```python
from build123d import *

# Parameters (mm, degrees)
SKETCH1_W                                   = 80
SKETCH1_H                                   = 60
BOSS_EXTRUDE1_DEPTH                         = 100
CUT_EXTRUDE1_START                          = 5
SKETCH2_W                                   = 35
SKETCH2_H                                   = 55
CUT_EXTRUDE1_DEPTH                          = 95
SKETCH3_W                                   = 80
SKETCH3_H                                   = 5
BOSS_EXTRUDE2_DEPTH                         = 70
BOSS_EXTRUDE3_DEPTH                         = 10
SKETCH5_W                                   = 22.5
SKETCH5_H                                   = 2.5
SKETCH5_W_2                                 = 20
CUT_EXTRUDE2_DEPTH                          = 7.5
SKETCH6_W                                   = 35
SKETCH6_H                                   = 12
CUT_EXTRUDE4_DEPTH                          = 57.5
CUT_EXTRUDE6_REACH                          = 184.483
SKETCH7_R                                   = 4
SKETCH9_W                                   = 80
SKETCH9_H                                   = 50
BOSS_EXTRUDE4_DEPTH                         = 5
SKETCH11_W                                  = 75
SKETCH11_H                                  = 32.5
CUT_EXTRUDE7_DEPTH                          = 2
SKETCH13_W                                  = 6
SKETCH13_H                                  = 6
CUT_EXTRUDE8_DEPTH                          = 166.90660023
BOSS_EXTRUDE5_DEPTH                         = 10
SKETCH15_W                                  = 6
SKETCH15_H                                  = 4
BOSS_EXTRUDE6_DEPTH                         = 1
BOSS_EXTRUDE7_START                         = -2.5
SKETCH15_2_W                                = 6
SKETCH15_2_H                                = 4
BOSS_EXTRUDE7_DEPTH                         = 1
SKETCH17_W                                  = 6
SKETCH17_H                                  = 4
BOSS_EXTRUDE8_DEPTH                         = 1
SKETCH18_W                                  = 3
SKETCH18_H                                  = 4
CUT_EXTRUDE9_OLED_CABLE_DEPTH               = 154.430766146
SKETCH20_W                                  = 5
SKETCH20_H                                  = 5
CUT_EXTRUDE10_SOLENOID_WIRE_DEPTH           = 166.90660023
SKETCH21_W                                  = 2
SKETCH21_H                                  = 32
BOSS_EXTRUDE9_SOLENOID_SIDE_SUPPORT_DEPTH   = 13
BOSS_EXTRUDE12_SOLENOID_REAR_SUPPORT_DEPTH  = 2
SKETCH27_W                                  = 2.5
SKETCH27_H                                  = 50
BOSS_EXTRUDE13_SOLENOID_SECTION_WALLS_DEPTH = 15
SKETCH29_W                                  = 70
SKETCH29_H                                  = 5
SKETCH29_W_2                                = 110
BOSS_EXTRUDE14_GUIDE_DEPTH                  = 5
BOSS_EXTRUDE15_START                        = -80
SKETCH29_2_W                                = 70
SKETCH29_2_H                                = 5
SKETCH29_2_W_2                              = 110
BOSS_EXTRUDE15_DEPTH                        = 5
SKETCH30_W                                  = 110
SKETCH30_H                                  = 2.5
SKETCH30_W_2                                = 70
BOSS_EXTRUDE16_DEPTH                        = 2.5
BOSS_EXTRUDE17_START                        = -87.5
SKETCH30_2_W                                = 110
SKETCH30_2_H                                = 2.5
SKETCH30_2_W_2                              = 70
BOSS_EXTRUDE17_DEPTH                        = 2.5


with BuildPart() as part:
    # Sketch1 → Boss-Extrude1 (new body)
    with BuildSketch(Plane(origin=(0, 0, 0), x_dir=(1, 0, 0), z_dir=(0, 1, 0))):
        with Locations((40, 30)):
            Rectangle(SKETCH1_W, SKETCH1_H)
    extrude(amount=BOSS_EXTRUDE1_DEPTH)

    # Sketch2 → Cut-Extrude1 (cut)
    with BuildSketch(Plane(origin=(0, 0, 0), x_dir=(1, 0, 0), z_dir=(0, 1, 0)).offset(CUT_EXTRUDE1_START)):
        with Locations((20, 30)):
            Rectangle(SKETCH2_W, SKETCH2_H)
        with Locations((60, 30)):
            Rectangle(SKETCH2_W, SKETCH2_H)
    extrude(amount=CUT_EXTRUDE1_DEPTH, mode=Mode.SUBTRACT)

    # Sketch3 → Boss-Extrude2 (add)
    with BuildSketch(Plane.XY):
        with Locations((40, 2.5)):
            Rectangle(SKETCH3_W, SKETCH3_H)
    extrude(amount=BOSS_EXTRUDE2_DEPTH)

    # Sketch4 → Boss-Extrude3 (add)
    with BuildSketch(Plane(origin=(0, 5, 0), x_dir=(1, 0, 0), z_dir=(0, 1, 0))):
        Polygon((80, 0), (77.5, 0), (77.5, -67.5), (42.5, -67.5), (42.5, 0), (37.5, 0), (37.5, -67.5), (2.5, -67.5), (2.5, 0), (0, 0), (0, -70), (80, -70), align=None)
    extrude(amount=BOSS_EXTRUDE3_DEPTH)

    # Sketch5 → Cut-Extrude2 (cut)
    with BuildSketch(Plane(origin=(0, 15, 0), x_dir=(1, 0, 0), z_dir=(0, 1, 0))):
        with Locations((18.75, -68.75)):
            Rectangle(SKETCH5_W, SKETCH5_H)
        with Locations((60, -68.75)):
            Rectangle(SKETCH5_W_2, SKETCH5_H)
    extrude(amount=-CUT_EXTRUDE2_DEPTH, mode=Mode.SUBTRACT)

    # Sketch6 → Cut-Extrude4 (cut)
    with BuildSketch(Plane.XY):
        with Locations((20, 11)):
            Rectangle(SKETCH6_W, SKETCH6_H)
        with Locations((60, 11)):
            Rectangle(SKETCH6_W, SKETCH6_H)
    extrude(amount=-CUT_EXTRUDE4_DEPTH, mode=Mode.SUBTRACT)

    # Sketch7 → Cut-Extrude6 (cut, up to next)
    with BuildSketch(Plane(origin=(0, 0, -60), x_dir=(-1, 0, 0), z_dir=(0, 0, -1)), mode=Mode.PRIVATE) as cut_extrude6_sk1:
        with Locations((-20, 11.5)):
            Circle(SKETCH7_R)
    cut_extrude6_tool1 = extrude(cut_extrude6_sk1.sketch, amount=-CUT_EXTRUDE6_REACH, mode=Mode.PRIVATE) & part.part
    # Sketch7 → Cut-Extrude6 (cut, up to next)
    with BuildSketch(Plane(origin=(0, 0, -60), x_dir=(-1, 0, 0), z_dir=(0, 0, -1)), mode=Mode.PRIVATE) as cut_extrude6_sk2:
        with Locations((-60, 11.5)):
            Circle(SKETCH7_R)
    cut_extrude6_tool2 = extrude(cut_extrude6_sk2.sketch, amount=-CUT_EXTRUDE6_REACH, mode=Mode.PRIVATE) & part.part
    add(cut_extrude6_tool1.solids().sort_by_distance((20, 11.5, -60))[0], mode=Mode.SUBTRACT)
    add(cut_extrude6_tool2.solids().sort_by_distance((60, 11.5, -60))[0], mode=Mode.SUBTRACT)

    # Sketch9 → Boss-Extrude4 (add)
    with BuildSketch(Plane(origin=(0, 0, 0), x_dir=(1, 0, 0), z_dir=(0, 1, 0))):
        with Locations((40, 85)):
            Rectangle(SKETCH9_W, SKETCH9_H)
    extrude(amount=BOSS_EXTRUDE4_DEPTH)

    # Sketch11 → Cut-Extrude7 (cut)
    with BuildSketch(Plane.XZ):
        with Locations((40, 53.75)):
            Rectangle(SKETCH11_W, SKETCH11_H)
    extrude(amount=-CUT_EXTRUDE7_DEPTH, mode=Mode.SUBTRACT)

    # Sketch13 → Cut-Extrude8 (cut, through all)
    with BuildSketch(Plane(origin=(0, 5, 0), x_dir=(1, 0, 0), z_dir=(0, 1, 0))):
        with Locations((20, -64.5)):
            Rectangle(SKETCH13_W, SKETCH13_H)
        with Locations((60, -64.5)):
            Rectangle(SKETCH13_W, SKETCH13_H)
    extrude(amount=-CUT_EXTRUDE8_DEPTH, mode=Mode.SUBTRACT)

    # Sketch14 → Boss-Extrude5 (add)
    with BuildSketch(Plane.XY):
        Polygon((25, 100), (26, 100), (26, 71), (54, 71), (54, 100), (55, 100), (55, 70), (54, 70), (26, 70), (25, 70), align=None)
    extrude(amount=BOSS_EXTRUDE5_DEPTH)

    # Sketch15 → Boss-Extrude6 (add)
    with BuildSketch(Plane.XY.offset(10)):
        with Locations((28, 72)):
            Rectangle(SKETCH15_W, SKETCH15_H)
        with Locations((52, 72)):
            Rectangle(SKETCH15_W, SKETCH15_H)
    extrude(amount=-BOSS_EXTRUDE6_DEPTH)

    # Sketch15<2> → Boss-Extrude7 (add)
    with BuildSketch(Plane.XY.offset(10).offset(BOSS_EXTRUDE7_START)):
        with Locations((28, 72)):
            Rectangle(SKETCH15_2_W, SKETCH15_2_H)
        with Locations((52, 72)):
            Rectangle(SKETCH15_2_W, SKETCH15_2_H)
    extrude(amount=-BOSS_EXTRUDE7_DEPTH)

    # Sketch17 → Boss-Extrude8 (add)
    with BuildSketch(Plane.XY.offset(10)):
        with Locations((28, 98)):
            Rectangle(SKETCH17_W, SKETCH17_H)
        with Locations((52, 98)):
            Rectangle(SKETCH17_W, SKETCH17_H)
    extrude(amount=-BOSS_EXTRUDE8_DEPTH)

    # Sketch18 → Cut-Extrude9 (OLED Cable) (cut, through all)
    with BuildSketch(Plane(origin=(0, 71, 0), x_dir=(1, 0, 0), z_dir=(0, 1, 0))):
        with Locations((40, -2)):
            Rectangle(SKETCH18_W, SKETCH18_H)
    extrude(amount=-CUT_EXTRUDE9_OLED_CABLE_DEPTH, mode=Mode.SUBTRACT)

    # Sketch20 → Cut-Extrude10 (Solenoid Wire) (cut, through all)
    with BuildSketch(Plane(origin=(0, 5, 0), x_dir=(1, 0, 0), z_dir=(0, 1, 0))):
        with Locations((60, 62.5)):
            Rectangle(SKETCH20_W, SKETCH20_H)
        with Locations((20, 62.5)):
            Rectangle(SKETCH20_W, SKETCH20_H)
    extrude(amount=-CUT_EXTRUDE10_SOLENOID_WIRE_DEPTH, mode=Mode.SUBTRACT)

    # Sketch21 → Boss-Extrude9 (Solenoid Side Support) (add)
    with BuildSketch(Plane(origin=(0, 5, 0), x_dir=(1, 0, 0), z_dir=(0, 1, 0))):
        with Locations((68.5, 76)):
            Rectangle(SKETCH21_W, SKETCH21_H)
        with Locations((51.5, 76)):
            Rectangle(SKETCH21_W, SKETCH21_H)
        with Locations((28.5, 76)):
            Rectangle(SKETCH21_W, SKETCH21_H)
        with Locations((11.5, 76)):
            Rectangle(SKETCH21_W, SKETCH21_H)
    extrude(amount=BOSS_EXTRUDE9_SOLENOID_SIDE_SUPPORT_DEPTH)

    # Sketch25 → Boss-Extrude12 (Solenoid Rear Support) (add)
    with BuildSketch(Plane(origin=(0, 0, -92), x_dir=(-1, 0, 0), z_dir=(0, 0, -1))):
        Polygon((-55.5, 18), (-52.5, 18), (-52.5, 15), align=None)
        Polygon((-52.5, 5), (-52.5, 8), (-55.5, 5), align=None)
        Polygon((-67.5, 18), (-67.5, 15), (-64.5, 18), align=None)
        Polygon((-64.5, 5), (-67.5, 5), (-67.5, 8), align=None)
        Polygon((-15.5, 18), (-12.5, 18), (-12.5, 15), align=None)
        Polygon((-12.5, 5), (-12.5, 8), (-15.5, 5), align=None)
        Polygon((-27.5, 18), (-27.5, 15), (-24.5, 18), align=None)
        Polygon((-24.5, 5), (-27.5, 5), (-27.5, 8), align=None)
    extrude(amount=-BOSS_EXTRUDE12_SOLENOID_REAR_SUPPORT_DEPTH)

    # Sketch27 → Boss-Extrude13 (Solenoid Section Walls) (add)
    with BuildSketch(Plane(origin=(0, 5, 0), x_dir=(1, 0, 0), z_dir=(0, 1, 0))):
        with Locations((78.75, 85)):
            Rectangle(SKETCH27_W, SKETCH27_H)
        with Locations((1.25, 85)):
            Rectangle(SKETCH27_W, SKETCH27_H)
    extrude(amount=BOSS_EXTRUDE13_SOLENOID_SECTION_WALLS_DEPTH)

    # Sketch29 → Boss-Extrude14 (Guide) (add)
    with BuildSketch(Plane(origin=(80, 0, 0), x_dir=(0, 0, -1), z_dir=(1, 0, 0))):
        with Locations((-35, 2.5)):
            Rectangle(SKETCH29_W, SKETCH29_H)
        with Locations((55, 15)):
            Rectangle(SKETCH29_W_2, SKETCH29_H)
    extrude(amount=BOSS_EXTRUDE14_GUIDE_DEPTH)

    # Sketch29<2> → Boss-Extrude15 (add)
    with BuildSketch(Plane(origin=(80, 0, 0), x_dir=(0, 0, -1), z_dir=(1, 0, 0)).offset(BOSS_EXTRUDE15_START)):
        with Locations((-35, 2.5)):
            Rectangle(SKETCH29_2_W, SKETCH29_2_H)
        with Locations((55, 15)):
            Rectangle(SKETCH29_2_W_2, SKETCH29_2_H)
    extrude(amount=-BOSS_EXTRUDE15_DEPTH)

    # Sketch30 → Boss-Extrude16 (add)
    with BuildSketch(Plane(origin=(85, 0, 0), x_dir=(0, 0, -1), z_dir=(1, 0, 0))):
        with Locations((55, 18.75)):
            Rectangle(SKETCH30_W, SKETCH30_H)
        with Locations((-35, 6.25)):
            Rectangle(SKETCH30_W_2, SKETCH30_H)
    extrude(amount=-BOSS_EXTRUDE16_DEPTH)

    # Sketch30<2> → Boss-Extrude17 (add)
    with BuildSketch(Plane(origin=(85, 0, 0), x_dir=(0, 0, -1), z_dir=(1, 0, 0)).offset(BOSS_EXTRUDE17_START)):
        with Locations((55, 18.75)):
            Rectangle(SKETCH30_2_W, SKETCH30_2_H)
        with Locations((-35, 6.25)):
            Rectangle(SKETCH30_2_W_2, SKETCH30_2_H)
    extrude(amount=-BOSS_EXTRUDE17_DEPTH)


solid = part.part
```
Can you work these out from the model? Positions are in its coordinate system, mm. A direction names the side the tool comes from. Give positions to 0.01 mm unless a question says otherwise; leave off trailing zeros. Write each loop counter-clockwise with the first axis right and the second up, starting at its lowest first coordinate (ties: lowest second). Pieces come first, ordered by that corner, then holes. Notation, with made-up numbers: (44.5, 47.5) -> (102.5, 47.5) arc R20 ccw to (102.5, 52.5) -> close; hole circle Ø6 at (84.25, 22.25). An arc over 180 degrees is marked (long way). One line per item, written item: value.
Q1. Imagine slicing it at A-A on x = 33. Please give me the cut outline in (y, z), and give its area (4 significant figures).
Results found:
outline: (0, -110) -> (5, -110) -> (5, -60) -> (100, -60) -> (100, -57.5) -> (5, -57.5) -> (5, 67.5) -> (15, 67.5) -> (15, 70) -> (2, 70) -> (2, 37.5) -> (0, 37.5) -> close; (17, -2.5) -> (100, -2.5) -> (100, 0) -> (71, 0) -> (71, 10) -> (70, 10) -> (70, 0) -> (17, 0) -> close
area: 1,315 mm^2
Q2. Imagine slicing it at D-D on x = 60. Please give me the cut outline in (y, z).
Results found:
outline: (0, -110) -> (5, -110) -> (5, -65) -> (0, -65) -> close; (0, -60) -> (7.5, -60) -> (7.5, -57.5) -> (5, -57.5) -> (5, 61.5) -> (2, 61.5) -> (2, 37.5) -> (0, 37.5) -> close; (2, 67.5) -> (7.5, 67.5) -> (7.5, 70) -> (2, 70) -> close; (15.5, -60) -> (100, -60) -> (100, -57.5) -> (15.5, -57.5) -> close; (17, -2.5) -> (100, -2.5) -> (100, 0) -> (17, 0) -> close
Q3. For P1, Ø0.8, axis at x = 81.5, z = 35, coming from the +Y side; P2, Ø0.8, axis at x = -3, z = -79.5, coming from the +Y side; P3, Ø8, axis at x = 60, z = 47, coming from the -Y side, each with a flat end and sliding along its axis, tell me the tip position at first contact or that it passes through.
Results found:
P1: stops at y = 5
P2: stops at y = 20
P3: stops at y = 2
Q4. Please list where these lines run through material, in increasing order: line 1 (X direction, y = 15, z = -51.5); line 2 (X direction, y = 59, z = -47); line 3 (Y direction, x = 60, z = -59). Write a range as [from, to].
Results found:
line 1: x = [-5, 2.5], [37.5, 42.5], [77.5, 85]
line 2: x = [0, 2.5], [37.5, 42.5], [77.5, 80]
line 3: y = [0, 7.5], [15.5, 100]
Q5. We'd pull the mould along Z, two halves only. Please class faces 1 (the face through (20, 3, -65)), 2 (the face through (41, 15, 40)), 3 (the face through (40.2, 4.8, -110)): +Z half, -Z half, draft (parallel to the pull), parting line (faces both ways), or undercut.
Results found:
face 1: undercut
face 2: draft
face 3: -Z half
Q6. Imagine slicing it at B-B on z = 53.5. Please give me the cut outline in (x, y), and give its area (4 significant figures).
Results found:
outline: (-5, 0) -> (2.5, 0) -> (2.5, 2) -> (77.5, 2) -> (77.5, 0) -> (85, 0) -> (85, 7.5) -> (82.5, 7.5) -> (82.5, 5) -> (80, 5) -> (80, 15) -> (77.5, 15) -> (77.5, 5) -> (42.5, 5) -> (42.5, 15) -> (37.5, 15) -> (37.5, 5) -> (2.5, 5) -> (2.5, 15) -> (0, 15) -> (0, 5) -> (-2.5, 5) -> (-2.5, 7.5) -> (-5, 7.5) -> close
area: 412.5 mm^2
Q7. Which directions (+Z, -Z, +X, -X, +Y, -Y) give clear straight access to the entire face, cutting with the end or side of a thin tool? Please do faces 4 (the face through (69.5, 11, -76)), 5 (the face through (20, 58, -2.5)), 6 (the face through (-2, 12.5, -54)).
Results found:
face 4: -Z, +Y
face 5: +Y
face 6: +Z, -Z, -X, -Y
Q8. Imagine slicing it at C-C on y = 32.5. Please give me the cut outline in (x, z), and give its area (3 significant figures).
Results found:
outline: (0, -60) -> (80, -60) -> (80, 0) -> (0, 0) -> close; hole (2.5, -57.5) -> (37.5, -57.5) -> (37.5, -2.5) -> (2.5, -2.5) -> close; hole (42.5, -57.5) -> (77.5, -57.5) -> (77.5, -2.5) -> (42.5, -2.5) -> close
area: 950 mm^2
